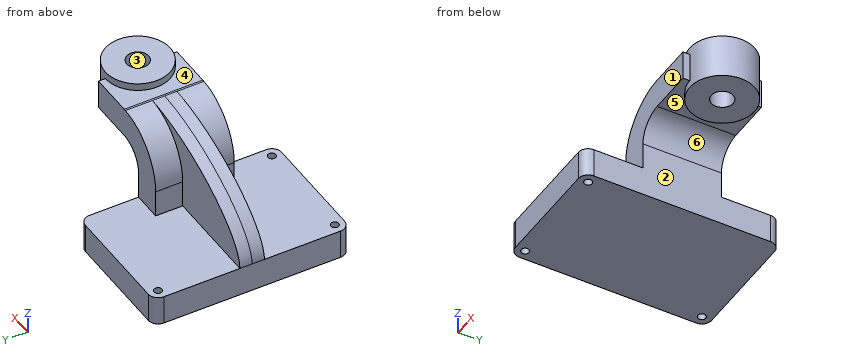
from build123d import *

# Parameters (mm, degrees)
F1_DEPTH  = 63.5
F2_DEPTH  = 25.4
F3_DEPTH  = 7.9375
F4_R      = 6.35
F6_R      = 7.0800960526
F7_DEPTH  = 34.544
F8_R      = 2.54
F9_DEPTH  = 25.4
F10_R     = 2.54
F11_DEPTH = 25.4
F12_DEPTH = 25.4


with BuildPart() as f1:
    # F0 (on Front) → F1 (new body, symmetric)
    with BuildSketch(Plane.XZ):
        Polygon((41.275, -9.525), (41.275, 9.525), (22.225, 9.525), (-41.275, 9.525), (-41.275, -9.525), align=None)
    extrude(amount=F1_DEPTH, both=True)

    # F0 (on Front) → F2 (join, symmetric)
    with BuildSketch(Plane.XZ):
        with BuildLine():
            Line((22.225, 9.525), (41.275, 9.525))
            Line((41.275, 9.525), (41.275, 27.0002))
            ThreePointArc((41.275, 27.0002), (45.4965819701, 37.7804353045), (55.9160674925, 42.827171775))
            Line((55.9160674925, 42.827171775), (55.9160674925, 61.9033952057))
            ThreePointArc((55.9160674925, 61.9033952057), (32.0218214167, 51.2557203219), (22.225, 27.0002))
            Line((22.225, 27.0002), (22.225, 9.525))
        make_face()
        with BuildLine():
            Line((55.9160674925, 61.9033952057), (55.9160674925, 42.827171775))
            ThreePointArc((55.9160674925, 42.827171775), (56.5325665737, 42.8631883995), (57.15, 42.8752))
            Line((57.15, 42.8752), (85.725, 42.8752))
            Line((85.725, 42.8752), (85.725, 61.9252))
            Line((85.725, 61.9252), (57.15, 61.9252))
            ThreePointArc((57.15, 61.9252), (56.5329374257, 61.9197483759), (55.9160674925, 61.9033952057))
        make_face()
    extrude(amount=F2_DEPTH, both=True)

    # F0 (on Front) → F3 (join, symmetric)
    with BuildSketch(Plane.XZ):
        with BuildLine():
            Line((-41.275, 9.525), (22.225, 9.525))
            Line((22.225, 9.525), (22.225, 27.0002))
            ThreePointArc((22.225, 27.0002), (32.0218214167, 51.2557203219), (55.9160674925, 61.9033952057))
            Line((55.9160674925, 61.9033952057), (55.9160674925, 61.9252))
            add(Edge.make_bspline(
                [(-41.275, 9.525), (-40.4172204435, 33.1299565732), (11.4771540301, 60.651878911), (55.9160674925, 61.9252)],
                knots=[0, 0, 0, 0, 110.4168671914, 110.4168671914, 110.4168671914, 110.4168671914], degree=3))
        make_face()
    extrude(amount=F3_DEPTH, both=True)

    # F4
    f4_edges = [f1.edges().sort_by_distance(p)[0] for p in [
        (41.275, -63.5, 0),
        (-41.275, -63.5, 0),
        (41.275, 63.5, 0),
        (-41.275, 63.5, 0),
    ]]
    fillet(f4_edges, radius=F4_R)

    # F0 (on Front) → F5 (revolve)
    with BuildSketch(Plane.XZ):
        Polygon((85.725, 42.8752), (85.725, 38.1), (106.7160674925, 38.1), (106.7160674925, 66.675), (85.725, 66.675), (85.725, 61.9252), align=None)
    revolve(axis=Axis((85.725, 0, 52.3875), (0, 0, -1)))

    # F6 (on face) → F7 (cut)
    with BuildSketch(Plane.XY.offset(66.675)):
        with Locations((85.725, 0)):
            Circle(F6_R)
    extrude(amount=-F7_DEPTH, mode=Mode.SUBTRACT)

    # F8 (on face) → F9 (cut)
    with BuildSketch(Plane.XY.offset(9.525)):
        with Locations((-34.925, -57.15)):
            Circle(F8_R)
    extrude(amount=-F9_DEPTH, mode=Mode.SUBTRACT)

    # F10 (on face) → F11 (cut)
    with BuildSketch(Plane.XY.offset(9.525)):
        with Locations((-34.925, 57.15)):
            Circle(F10_R)
    extrude(amount=-F11_DEPTH, mode=Mode.SUBTRACT)

    # F8 (on face) → F12 (cut)
    with BuildSketch(Plane.XY.offset(9.525)):
        with Locations((34.925, -57.15)):
            Circle(F8_R)
    extrude(amount=-F12_DEPTH, mode=Mode.SUBTRACT)


solid = f1.part
Can you work these out from the model? Positions are in its coordinate system, mm. Face numbers are marked on the shaded views. A direction names the side the tool comes from. Coordinates: 2 decimals unless noted, no trailing zeros. Write each loop counter-clockwise with the first axis right and the second up, starting at its lowest first coordinate (ties: lowest second). Pieces come first, ordered by that corner, then holes.
Q1. Which directions (+Z, -Z, +X, -X, +Y, -Y) give clear straight access to the entire face, cutting with the end or side of a thin tool? Please do the marked faces 4, 5 and 6.
Results found:
face 4: +Z, -X
face 5: -Z
face 6: -Z, +Y, -Y
Q2. Please list where these lines run through material, in increasing order: L1, parallel to X at y = -57, z = 5 (3 decimals); L2, parallel to X at y = 4, z = -5 (3 decimals); L3, parallel to Y at x = 18.5, z = 15.
Results found:
L1: x = -41.275 to -37.461, -32.389 to 32.389, 37.461 to 41.275
L2: x = -41.275 to 41.275
L3: y = -7.94 to 7.94
Q3. If we mould it in two halves opening along Y, with no side actions, what happens to the marked faces 1, 2 and 3? For each: +Y half, -Y half, draft (parallel to the pull), parting line (faces both ways), or undercut.
Results found:
face 1: -Y half
face 2: draft
face 3: undercut
Q4. Imagine slicing it at C-C, the plane y = -29. List the corners of the cut face in (x, z) for me (3 decimals).
Results found:
outline: (-41.275, -9.525) - (41.275, -9.525) - (41.275, 9.525) - (-41.275, 9.525) - close
Q5. Imagine slicing it at A-A, the plane z = -3. List the corners of the cut face in (x, y) for me (3 decimals).
Results found:
outline: (-41.275, -57.15) arc R6.35 ccw to (-34.925, -63.5) - (34.925, -63.5) arc R6.35 ccw to (41.275, -57.15) - (41.275, 57.15) arc R6.35 ccw to (34.925, 63.5) - (-34.925, 63.5) arc R6.35 ccw to (-41.275, 57.15) - close; hole circle Ø5.08 at (-34.925, -57.15); hole circle Ø5.08 at (-34.925, 57.15); hole circle Ø5.08 at (34.925, -57.15)
Q6. For P1, Ø8, axis at x = -34.925, y = -57.15, coming from the +Z side (3 decimals); P2, Ø14, axis at y = -20, z = 21.5, coming from the -X side (3 decimals); P3, Ø2, axis at y = 24, z = 52.5, coming from the +X side (3 decimals), each with a flat end and sliding along its axis, tell me the tip position at first contact or that it passes through.
Results found:
P1: stops at z = 9.525
P2: stops at x = 22.225
P3: stops at x = 85.725
Q7. Imagine slicing it at B-B, the plane y = -12.5. List the corners of the cut face in (x, z) for me (3 decimals), plus the area to 3 significant figures.
Results found:
outline: (-41.275, -9.525) - (41.275, -9.525) - (41.275, 27) arc R15.875 cw to (57.15, 42.875) - (68.862, 42.875) - (68.862, 38.1) - (102.588, 38.1) - (102.588, 66.675) - (68.862, 66.675) - (68.862, 61.925) - (57.15, 61.925) arc R34.925 ccw to (22.225, 27) - (22.225, 9.525) - (-41.275, 9.525) - close
area: 3,850 mm2
